Source: CAD feature listing. Evaluate the final solid. Frame: model axes, mm. A direction names the side the tool comes from. Give positions to 0.01 mm unless a question says otherwise; leave off trailing zeros. Loops run counter-clockwise (first coordinate to the right, second up) from the corner with the lowest first, then second, coordinate; pieces in that order, holes last.
from build123d import *

# Parameters (mm, degrees)
F0_W      = 1000
F0_H      = 530
F1_DEPTH  = 30
F2_R      = 3
F3_DEPTH  = 12
F4_R      = 3
F5_DEPTH  = 12
F7_R      = 3
F8_DEPTH  = 12
F9_R      = 3
F10_DEPTH = 12
F6_R      = 250
F11_DEPTH = 15
F12_R     = 3
F13_DEPTH = 5
F14_R     = 3
F15_DEPTH = 12


with BuildPart() as f1:
    # F0 (on Top) → F1 (new body)
    with BuildSketch(Plane.XY):
        with Locations((500, 265)):
            Rectangle(F0_W, F0_H)
    extrude(amount=F1_DEPTH)

    # F2 (on face) → F3 (cut)
    with BuildSketch(Plane(origin=(0, 0, 0), x_dir=(1, 0, 0), z_dir=(0, 0, -1))):
        with Locations((985, -130)):
            Circle(F2_R)
    extrude(amount=-F3_DEPTH, mode=Mode.SUBTRACT)

    # F4 (on face) → F5 (cut)
    with BuildSketch(Plane(origin=(0, 0, 0), x_dir=(1, 0, 0), z_dir=(0, 0, -1))):
        with Locations((15, -130)):
            Circle(F4_R)
    extrude(amount=-F5_DEPTH, mode=Mode.SUBTRACT)

    # F7 (on face) → F8 (cut)
    with BuildSketch(Plane(origin=(0, 0, 0), x_dir=(1, 0, 0), z_dir=(0, 0, -1))):
        with Locations((985, -400)):
            Circle(F7_R)
    extrude(amount=-F8_DEPTH, mode=Mode.SUBTRACT)

    # F9 (on face) → F10 (cut)
    with BuildSketch(Plane(origin=(0, 0, 0), x_dir=(1, 0, 0), z_dir=(0, 0, -1))):
        with Locations((15, -400)):
            Circle(F9_R)
    extrude(amount=-F10_DEPTH, mode=Mode.SUBTRACT)

    # F6 (on face) → F11 (cut)
    with BuildSketch(Plane.XY.offset(30)):
        with Locations((500, 265)):
            Circle(F6_R)
    extrude(amount=-F11_DEPTH, mode=Mode.SUBTRACT)

    # F12 (on face) → F13 (cut)
    with BuildSketch(Plane.XY.offset(15)):
        with Locations((500, 265)):
            Circle(F12_R)
    extrude(amount=-F13_DEPTH, mode=Mode.SUBTRACT)

    # F14 (on face) → F15 (cut)
    with BuildSketch(Plane(origin=(0, 0, 0), x_dir=(1, 0, 0), z_dir=(0, 0, -1))):
        with Locations((500, -515)):
            Circle(F14_R)
    extrude(amount=-F15_DEPTH, mode=Mode.SUBTRACT)


solid = f1.part
1) Ray query, probe 1 along Y at (x, z) = (985, 6); probe 2 along X at (y, z) = (400, 3); probe 3 along X at (y, z) = (265, 11.3). Return the intervals inside material, ascending.
Checks:
probe 1: y = 0 to 127, 133 to 397, 403 to 530
probe 2: x = 0 to 12, 18 to 982, 988 to 1000
probe 3: x = 0 to 497, 503 to 1000
2) Cut plane B-B (z = 20). Return loops of the section in (x, y), and give its area (3 significant figures).
Checks:
outline: (0, 0) - (1000, 0) - (1000, 530) - (0, 530) - close; hole circle Ø500 at (500, 265)
area: 334,000 mm2
3) Reachability of faces 1 (the flat face through (271, 151, 30)), 2 (the cylindrical face through (730.936, 169.249, 22.605)) from +Z, -Z, +X, -X, +Y, -Y: full face, straight path, thin tool, end or side. Return the list, or none.
Checks:
face 1: +Z, +X, -X, +Y, -Y
face 2: +Z
4) Cut plane A-A (x = 562). Return loops of the section in (y, z).
Checks:
outline: (0, 0) - (530, 0) - (530, 30) - (507.19, 30) - (507.19, 15) - (22.81, 15) - (22.81, 30) - (0, 30) - close
5) Cut plane C-C (y = 117). Return loops of the section in (x, z), and give its area (3 significant figures).
Checks:
outline: (0, 0) - (1000, 0) - (1000, 30) - (701.48, 30) - (701.48, 15) - (298.52, 15) - (298.52, 30) - (0, 30) - close
area: 24,000 mm2
6) Contact query for flat-ended pins moving along their axis: P1, Ø1.8, axis at x = 500.5, y = 265, coming from the +Z side; P2, Ø1.8, axis at x = 499, y = 515, coming from the -Z side; P3, Ø2, axis at x = 319, y = 423.5, coming from the +Z side. Output: stop coordinate, or through.
Checks:
P1: stops at z = 10
P2: stops at z = 12
P3: stops at z = 15
7) Pull-direction query (Y, two-part tool) for faces 3 (the flat face through (496, 268, 15)), 4 (the flat face through (493, 530, 15)), 5 (the flat face through (0, 261, 15)); classes: released by +Y, released by -Y, zero draft, split by the parting line, or undercut.
Checks:
face 3: undercut
face 4: released by +Y
face 5: zero draft
